from build123d import *

# Parameters (mm, degrees)
BOSS_EXTRUDE1_DEPTH     = 4
CUT_EXTRUDE1_DEPTH      = 5
CUT_EXTRUDE1_DEPTH_BACK = 1
SKETCH1_6_R             = 10
CUT_EXTRUDE2_DEPTH      = 1.93
CUT_EXTRUDE2_DEPTH_BACK = 1
M2_5_CLEARANCE_HOLE1_D  = 2.9
CHAMFER1_SIZE           = 0.25


with BuildPart() as part:
    # Sketch1 → Boss-Extrude1 (new body)
    with BuildSketch(Plane.XY):
        with BuildLine():
            ThreePointArc((16.285714286, -3.282607227), (18, 0), (16.285714286, 3.282607227))
            Line((16.285714286, 3.282607227), (6.857142857, 9.84782168))
            ThreePointArc((6.857142857, 9.84782168), (0, 12), (-6.857142857, 9.84782168))
            Line((-6.857142857, 9.84782168), (-16.285714286, 3.282607227))
            ThreePointArc((-16.285714286, 3.282607227), (-18, 0), (-16.285714286, -3.282607227))
            Line((-16.285714286, -3.282607227), (-6.857142857, -9.84782168))
            ThreePointArc((-6.857142857, -9.84782168), (0, -12), (6.857142857, -9.84782168))
            Line((6.857142857, -9.84782168), (16.285714286, -3.282607227))
        make_face()
    extrude(amount=BOSS_EXTRUDE1_DEPTH)

    # Sketch1_4 → Cut-Extrude1 (cut, two sides)
    with BuildSketch(Plane.XY) as cut_extrude1_sk:
        with BuildLine():
            ThreePointArc((-8.25, 0), (0, -8.25), (8.25, 0))
            Line((8.25, 0), (-8.25, 0))
        make_face()
        with BuildLine():
            Line((-8.25, 0), (8.25, 0))
            ThreePointArc((8.25, 0), (0, 8.25), (-8.25, 0))
        make_face()
    extrude(amount=CUT_EXTRUDE1_DEPTH, mode=Mode.SUBTRACT)
    extrude(cut_extrude1_sk.sketch, amount=-CUT_EXTRUDE1_DEPTH_BACK, mode=Mode.SUBTRACT)

    # Sketch1_6 → Cut-Extrude2 (cut, two sides)
    with BuildSketch(Plane.XY) as cut_extrude2_sk:
        Circle(SKETCH1_6_R)
    extrude(amount=CUT_EXTRUDE2_DEPTH, mode=Mode.SUBTRACT)
    extrude(cut_extrude2_sk.sketch, amount=-CUT_EXTRUDE2_DEPTH_BACK, mode=Mode.SUBTRACT)

    # M2.5 Clearance Hole1 (through all)
    with Locations(Plane.XY.offset(4)):
        with Locations((-14, 0), (14, 0)):
            Hole(M2_5_CLEARANCE_HOLE1_D / 2)

    # Chamfer1
    chamfer1_edges = [part.edges().sort_by_distance(p)[0] for p in [
        (-18, 0, 4),
        (-11.571428571, -6.565214453, 4),
        (11.571428571, 6.565214453, 4),
        (18, 0, 4),
        (11.571428571, -6.565214453, 4),
        (0, 12, 4),
        (0, -12, 4),
        (-8.25, 0, 4),
        (-10, 0, 0),
        (-10, 0, 1.93),
        (-8.25, 0, 1.93),
        (-11.571428571, 6.565214453, 4),
    ]]
    chamfer(chamfer1_edges, length=CHAMFER1_SIZE)


solid = part.part
The listing builds one solid part. Answer for the finished solid, in the listing's coordinates (mm). A direction names the side the tool comes from. Round coordinates to 2 decimals unless told otherwise and drop trailing zeros. Loops run counter-clockwise (first coordinate to the right, second up) from the corner with the lowest first, then second, coordinate; pieces in that order, holes last. Notation, with made-up numbers: M 6,71 L 17,71 A22 cw 17,81 Z; hole C -40,-22.75 d1. An arc over 180 degrees is marked long. Write each question's results on one line, items separated by ' | '. Start each with the question number.
1) Find section A-A on x = 0. Write down the section's boundary in (y, z).
2) Determine the mould class of faces 3 (the conical face through (-17.88, 0.05, 3.87)), 4 (the conical face through (0.1, 11.88, 3.87)), 5 (the cylindrical face through (-15.339, -0.555, 1.972)) for opening direction X: pulls with the +X half, pulls with the -X half, needs draft (parallel to the pull), parting line crosses it, or undercut.
3) Find section C-C on z = 0.8. Write down the section's boundary in (x, y), plus the area to 3 significant figures.
4) Find section D-D on x = -13. Write down the section's boundary in (y, z).
5) Find section B-B on y = 0. Count the separate pieces of the cut face and the enclosed holes in it, plus the area to 3 significant figures.
6) Straight lines are drawn through the part: probe 1 along X at (y, z) = (-1, 3.55); probe 2 along Y at (x, z) = (-7, 3.2); probe 3 along X at (y, z) = (-4.75, 2.2). For each, find the intervals that lie inside material, in ascending order.
7) Which of the six approach directions +Z, -Z, +X, -X, +Y, -Y give full straight-line access (tool end or side, diameter ignored) to faces 1 (the cylindrical face through (18, 0, 2)), 2 (the cylindrical face through (-2.17, -9.76, 0.95))?
8) Each of these flat-tipped pins is pushed along its axis until it touches: pin 1 (1.7 mm diameter, centred on x = -14, y = 0, fed in from +Z); pin 2 (1.5 mm diameter, centred on y = 1, z = 0.5, fed in from -X); pin 3 (1 mm diameter, centred on y = 8, z = 0.5, fed in from +X). Where does it stop, or does it pass through?
Final values:
1) outline: M -12,0 L -10.25,0 L -10,0.25 L -10,1.68 L -9.75,1.93 L -8.5,1.93 L -8.25,2.18 L -8.25,3.75 L -8.5,4 L -11.75,4 L -12,3.75 Z; M 8.25,2.18 L 8.5,1.93 L 9.75,1.93 L 10,1.68 L 10,0.25 L 10.25,0 L 12,0 L 12,3.75 L 11.75,4 L 8.5,4 L 8.25,3.75 Z
2) face 3: pulls with the -X half | face 4: parting line crosses it | face 5: undercut
3) outline: M -16.29,-3.28 L -6.86,-9.85 A12 ccw 6.86,-9.85 L 16.29,-3.28 A4 ccw 16.29,3.28 L 6.86,9.85 A12 ccw -6.86,9.85 L -16.29,3.28 A4 ccw Z; hole C -14,0 d2.9; hole C 0,0 d20; hole C 14,0 d2.9 | area: 246 mm²
4) outline: M -5.57,0 L -1.05,0 L -1.05,4 L -5.27,4 L -5.57,3.75 Z; M 1.05,0 L 5.57,0 L 5.57,3.75 L 5.27,4 L 1.05,4 Z
5) separate pieces: 4 | enclosed holes: 0 | area: 47.9 mm²
6) probe 1: -17.87 to -15.05, -12.95 to -8.19, 8.19 to 12.95, 15.05 to 17.87 | probe 2: -9.75 to -4.37, 4.37 to 9.75 | probe 3: -14.18 to -6.75, 6.75 to 14.18
7) face 1: +Z, -Z, +X | face 2: -Z
8) pin 1: through | pin 2: x = -17.99 | pin 3: x = 10.23
